Design review of the part shown in the three views and the two pictorial views. Dimensions are in mm from the part's minimum x, y and z. A direction names the side the tool comes from. Round coordinates to 2 decimals unless told otherwise and drop trailing zeros. Order: outer loops, then holes, each group sorted by start corner. A loop starts at its lowest first (then second) coordinate and runs counter-clockwise, first axis right, second up. Notation, with made-up numbers: M 56,-19 L 114,-19 A7 ccw 114,-8 Z; hole C -29.5,1 d10. An arc over 180 degrees is marked long. Use a Markdown table: item, result. Add a question column.
(1) For pin 1 (4.5 mm diameter, centred on x = 7.5, y = 8, fed in from -Z); pin 2 (1.5 mm diameter, centred on y = 16, z = 8, fed in from +X); pin 3 (1.8 mm diameter, centred on x = 8, y = 14.9, fed in from +Z), all flat-tipped, find the tip position at first contact; note any pin that passes through.
(2) To check wall thickness, follow probe 1 along Y at (x, z) = (0.75, 2); probe 2 along Y at (x, z) = (8, 9.55); probe 3 along X at (y, z) = (14.5, 0.5). State the ranges of each line that lie inside material, in increasing order. Write a range as from..to.
(3) Take a section at D-D (z = 8.75). Write out the cut boundary in (x, y), then the cut area to 3 significant figures.
(4) Machinability: for the marked faces 1 and 2, which of the approach directions +Z, -Z, +X, -X, +Y, -Y give a long, thin tool a straight path to every point of the face, cutting with its end or side? Answer none if there is none.
(5) Take a section at C-C (y = 6.5). Write out the cut boundary in (x, z), then the cut area to 3 significant figures.
(6) Take a section at B-B (x = 8). Write out the cut boundary in (y, z).
(7) Take a section at A-A (z = 2). Write out the cut boundary in (x, y).
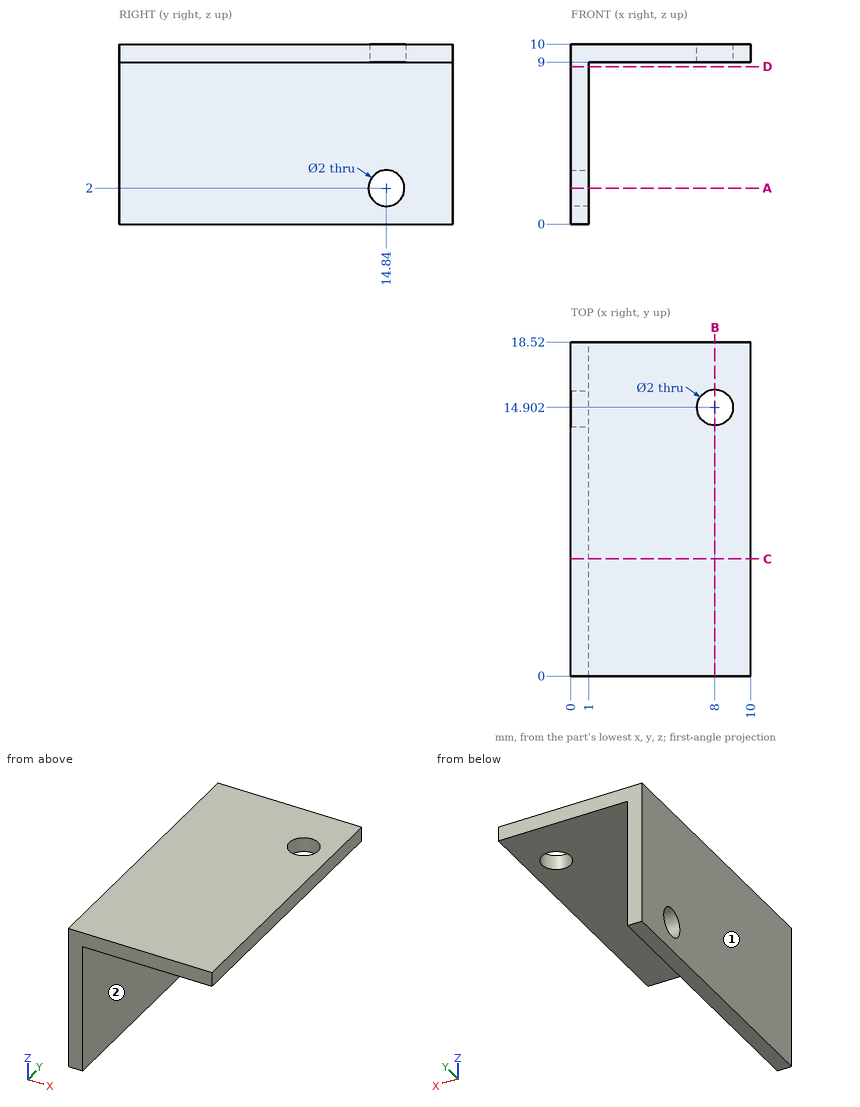
Verdict:
| question | item | result |
|---|---|---|
| 1 | pin 1 | stops at z = 9 |
| 1 | pin 2 | stops at x = 1 |
| 1 | pin 3 | passes through |
| 2 | probe 1 | y = 0..13.84, 15.84..18.52 |
| 2 | probe 2 | y = 0..13.9, 15.9..18.52 |
| 2 | probe 3 | x = 0..1 |
| 3 | outline | M 0,0 L 1,0 L 1,18.52 L 0,18.52 Z |
| 3 | area | 18.5 mm^2 |
| 4 | face 1 | +Z, -Z, -X, +Y, -Y |
| 4 | face 2 | -Z, +X, +Y, -Y |
| 5 | outline | M 0,0 L 1,0 L 1,9 L 10,9 L 10,10 L 0,10 Z |
| 5 | area | 19.0 mm^2 |
| 6 | outline | M 0,9 L 13.9,9 L 13.9,10 L 0,10 Z; M 15.9,9 L 18.52,9 L 18.52,10 L 15.9,10 Z |
| 7 | outline | M 0,0 L 1,0 L 1,13.84 L 0,13.84 Z; M 0,15.84 L 1,15.84 L 1,18.52 L 0,18.52 Z |
